Work out the finished part from the listing and answer in its coordinate system (mm). A direction names the side the tool comes from. Coordinates: 2 decimals unless noted, no trailing zeros. Order: outer loops, then holes, each group sorted by start corner. A loop starts at its lowest first (then second) coordinate and runs counter-clockwise, first axis right, second up.
1. A tool of negligible diameter and unlimited length cuts with its end or side. For faces 1 (the flat face through (0, 3, 5)), 2 (the flat face through (19, 1, -2)), 3 (the cylindrical face through (2.86, -0.9, -2.46)), from which of +Z, -Z, +X, -X, +Y, -Y can it reach the whole face along a straight path? Write none if from no direction.
2. The part is cut by section C-C, the plane x = -22. Give the vertices of the cut face in (y, z).
3. The part is cut by section B-B, the plane y = 6. Give the vertices of the cut face in (x, z), then the cut area to 3 significant figures.
4. The part is cut by section A-A, the plane z = -1. Give the vertices of the cut face in (x, y), then the cut area to 3 significant figures.
5. Flat-ended cylindrical pins translate along their axes: pin 1 Ø1.9 at (x, y) = (0, 0) entering from -Z; pin 2 Ø5 at (x, y) = (-6.5, 1) entering from -Z. Find the tip coordinate at first contact, or state that the pin passes through.
6. Determine the mould class of faces 4 (the cylindrical face through (-22.74, 4.58, 0.07)), 5 (the flat face through (25, 1, 0)), 6 (the flat face through (-22, 1, -5)) for opening direction X: +X half, -X half, draft (parallel to the pull), parting line (faces both ways), or undercut.
7. The part is cut by section D-D, the plane y = 1. Give the vertices of the cut face in (x, z).
8. Find the intervals of material crossed by probe 1 along Y at (x, z) = (-22, -3); probe 2 along Y at (x, z) = (-11, 2.75); probe 3 along X at (y, z) = (5.75, 0.5), in increasing order.
```python
from build123d import *

# Parameters (mm, degrees)
SKETCH1_W               = 50
SKETCH1_H               = 16
BOSS_EXTRUDE1_DEPTH     = 5
SKETCH2_R               = 3
SKETCH2_W               = 6
SKETCH2_H               = 16
BOSS_EXTRUDE2_DEPTH     = 5
CUT_EXTRUDE1_DEPTH      = 28.037011669
CUT_EXTRUDE1_DEPTH_BACK = 28.037011669
SKETCH3_R               = 1.6


with BuildPart() as part:
    # Sketch1 → Boss-Extrude1 (new body)
    with BuildSketch(Plane.XY):
        with Locations((0, 1)):
            Rectangle(SKETCH1_W, SKETCH1_H)
    extrude(amount=BOSS_EXTRUDE1_DEPTH)

    # Sketch2 → Boss-Extrude2 (add)
    with BuildSketch(Plane(origin=(0, 0, 0), x_dir=(-1, 0, 0), z_dir=(0, 0, -1))):
        with Locations(Location((0, 0, 0), (0, 0, 180))):
            Circle(SKETCH2_R)
        with Locations((22, 1)):
            Rectangle(SKETCH2_W, SKETCH2_H)
        with Locations((-22, 1)):
            Rectangle(SKETCH2_W, SKETCH2_H)
    extrude(amount=BOSS_EXTRUDE2_DEPTH)

    # Sketch3 → Cut-Extrude1 (cut, two sides: drawn at the far end of the back side and taken through both)
    with BuildSketch(Plane(origin=(0, 0, 0), x_dir=(-1, 0, 0), z_dir=(0, 0, -1)).offset(-CUT_EXTRUDE1_DEPTH_BACK)):
        Circle(SKETCH3_R)
        with Locations((11, 0)):
            Circle(SKETCH3_R)
        with Locations((22, -4)):
            Circle(SKETCH3_R)
        with Locations((22, 6)):
            Circle(SKETCH3_R)
        with Locations(Location((-22, 6, 0), (0, 0, 180))):
            Circle(SKETCH3_R)
        with Locations(Location((-22, -4, 0), (0, 0, 180))):
            Circle(SKETCH3_R)
        with Locations(Location((-11, 0, 0), (0, 0, 180))):
            Circle(SKETCH3_R)
    extrude(amount=CUT_EXTRUDE1_DEPTH + CUT_EXTRUDE1_DEPTH_BACK, mode=Mode.SUBTRACT)


solid = part.part
```
Geometry says:
1. face 1: +Z, +X, -X, +Y, -Y
1. face 2: -Z, +Y, -Y
1. face 3: -Z
2. outline: (-7, -5) - (-5.6, -5) - (-5.6, 5) - (-7, 5) - close; (-2.4, -5) - (4.4, -5) - (4.4, 5) - (-2.4, 5) - close; (7.6, -5) - (9, -5) - (9, 5) - (7.6, 5) - close
3. outline: (-25, -5) - (-23.6, -5) - (-23.6, 5) - (-25, 5) - close; (-20.4, -5) - (-19, -5) - (-19, 0) - (19, 0) - (19, -5) - (20.4, -5) - (20.4, 5) - (-20.4, 5) - close; (23.6, -5) - (25, -5) - (25, 5) - (23.6, 5) - close
3. area: 246 mm2
4. outline: (-25, -7) - (-19, -7) - (-19, 9) - (-25, 9) - close; circle Ø6 at (0, 0); (19, -7) - (25, -7) - (25, 9) - (19, 9) - close; hole circle Ø3.2 at (-22, -4); hole circle Ø3.2 at (-22, 6); hole circle Ø3.2 at (0, 0); hole circle Ø3.2 at (22, -4); hole circle Ø3.2 at (22, 6)
4. area: 180 mm2
5. pin 1: passes through
5. pin 2: stops at z = 0
6. face 4: undercut
6. face 5: +X half
6. face 6: draft
7. outline: (-25, -5) - (-19, -5) - (-19, 0) - (-12.25, 0) - (-12.25, 5) - (-25, 5) - close; (-9.75, 0) - (-2.83, 0) - (-2.83, -5) - (-1.25, -5) - (-1.25, 5) - (-9.75, 5) - close; (1.25, -5) - (2.83, -5) - (2.83, 0) - (9.75, 0) - (9.75, 5) - (1.25, 5) - close; (12.25, 0) - (19, 0) - (19, -5) - (25, -5) - (25, 5) - (12.25, 5) - close
8. probe 1: y = -7 to -5.6, -2.4 to 4.4, 7.6 to 9
8. probe 2: y = -7 to -1.6, 1.6 to 9
8. probe 3: x = -25 to -23.58, -20.42 to 20.42, 23.58 to 25
